Geometry check sheet. Reference: the model listing, model coordinates, mm. Face numbers are marked on the shaded views. A direction names the side the tool comes from. Give positions to 0.01 mm unless a question says otherwise; leave off trailing zeros. Write each loop counter-clockwise with the first axis right and the second up, starting at its lowest first coordinate (ties: lowest second). Pieces come first, ordered by that corner, then holes.
(1) Tool access check on the marked faces 1, 2, 3 and 4. Record the directions out of +Z, -Z, +X, -X, +Y, -Y that give a thin tool (end or side, any length) a straight path to the whole face; none if there is none.
(2) Cross-section at D-D (z = -2.5). Record the boundary of the cut face in (x, y) (3 decimals), and give its area (3 significant figures).
(3) Cross-section at C-C (y = -7.75). Record the boundary of the cut face in (x, z) (3 decimals).
(4) Cross-section at B-B (x = -2.4). Record the boundary of the cut face in (y, z) (3 decimals).
(5) Mould release check, pull along Z, two halves, no side actions. Record for the marked faces 5, 6 and 7: +Z half, -Z half, draft (parallel to the pull), parting line (faces both ways), or undercut.
(6) Thickness scan on line 1 along Z through (x, y) = (-2.5, -11) (3 decimals); line 2 along Z through (x, y) = (-13.6, -10.35) (3 decimals); line 3 along Z through (x, y) = (-5, -10.25) (3 decimals). Record the ranges inside material, lowest first.
(7) Depth check by flat-ended pin: P1, Ø1.3, axis at x = -8.5, y = 3.5, coming from the -Z side (3 decimals); P2, Ø5.5, axis at x = -13.6, z = 16.675, coming from the -Y side; P3, Ø2, axis at y = -1, z = -0.5, coming from the +X side; P4, Ø1, axis at x = -14.5, y = 2, coming from the +Z side (3 decimals). Enter the tip coordinate at first touch or a pass-through.
(8) Cross-section at A-A (y = -10.25). Record the boundary of the cut face in (x, z) (3 decimals).
Autodesk Inventor part; units mm, degrees
ref_plane "YZ Plane" through (0, 0, 0) normal (1, 0, 0) x (0, 1, 0)
ref_plane "XZ Plane" through (0, 0, 0) normal (0, 1, 0) x (-1, 0, 0)
ref_plane "XY Plane" through (0, 0, 0) normal (0, 0, 1) x (1, 0, 0)
sketch "Sketch1" plane through (0, 0, 0) normal (1, 0, 0) x (0, 1, 0)
  line L0 (2.5, 8) -> (-2.5, -8) construction
  line L1 (-2.5, 8) -> (2.5, -8) construction
  line L2 (2.5, 8) -> (2.5, 3.55)
  line L3 (2.5, -8) -> (2.5, -3.55)
  line L4 (-2.5, 0) -> (0.675, 0)
  line L5 (2.5, 8) -> (8.85, 8)
  line L6 (8.85, 8) -> (8.85, -8)
  line L7 (8.85, -8) -> (2.5, -8)
  arc A0 (2.5, -3.55) -> (2.5, 3.55) centre (0.675, 0) ccw
  line L8 (2.5, -8) -> (2.5, -3.55)
  line L9 (2.5, 3.55) -> (2.5, 8)
  point P0 (0, 0)
  dimension "d0" = 5
  dimension "d1" = 16
  dimension "d2" = 4.45
  dimension "d4" = 3.175
  dimension "d7" = 6.35
extrude "Extrusion1" add sketch "Sketch1" along normal blind 3.175
sketch "Sketch2" plane through (0, 0, 0) normal (-1, 0, 0) x (0, 0, 1)
  line L0 (-8, 8.85) -> (8, 8.85)
  line L1 (8, 2.5) -> (3.55, 2.5)
  line L2 (-8, 8.85) -> (8, 8.85)
  line L3 (8, 8.85) -> (8, 2.5)
  line L4 (8, 2.5) -> (-8, 2.5)
  line L5 (-8, 2.5) -> (-8, 8.85)
  point P0 (0, 0)
extrude "Extrusion2" add sketch "Sketch2" along normal blind 16
sketch "Sketch3" plane through (-16, 0, 0) normal (-1, 0, 0) x (0, 0, 1)
  line L0 (-8, 2.5) -> (-8, 8.85)
  line L1 (8, 2.5) -> (3.55, 2.5)
  line L2 (-8, 8.85) -> (8, 8.85)
  line L3 (8, 8.85) -> (8, 2.5)
  line L4 (8, 2.5) -> (-8, 2.5)
  line L5 (-8, 2.5) -> (-8, 8.85)
  point P0 (0, 0)
extrude "Extrusion3" add sketch "Sketch3" along normal blind 3.175
sketch "Sketch4" plane through (3.175, 2.5, 3.55) normal (0, -1, 0) x (1, 0, 0)
  line L0 (-22.35, -11.55) -> (-22.35, 4.45)
  line L1 (-3.175, -7.1) -> (0, -7.1)
  line L2 (-19.175, 0) -> (-3.175, 0)
  line L3 (-3.175, 0) -> (-3.175, -7.1)
  line L4 (-3.175, -7.1) -> (-19.175, -7.1)
  line L5 (-19.175, -7.1) -> (-19.175, 0)
  line L6 (-19.175, 0) -> (-3.175, -7.1) construction
  line L7 (-3.175, 0) -> (-19.175, -7.1) construction
  point P0 (-3.175, -3.55)
extrude "Extrusion4" cut sketch "Sketch4" against normal through all
sketch "Sketch5" plane through (-16, 2.5, 3.55) normal (1, 0, 0) x (0, 0, -1)
  line L0 (0, 6.35) -> (7.1, 6.35)
  line L1 (0, 0) -> (7.1, 0)
  line L2 (7.1, 0) -> (7.1, 6.35)
  line L3 (7.1, 6.35) -> (0, 6.35)
  line L4 (0, 6.35) -> (0, 0)
  point P0 (3.55, -2.5)
extrude "Extrusion5" cut sketch "Sketch5" against normal blind 0.25
sketch "Sketch6" plane through (0, 0.675, 0) normal (-1, 0, 0) x (0, 0, 1)
  line L0 (-3.55, 1.825) -> (-3.55, 8.175)
  line L1 (3.55, 1.825) -> (3.55, 8.175)
  line L2 (-3.55, 1.825) -> (3.55, 1.825)
  line L3 (3.55, 1.825) -> (3.55, 8.175)
  line L4 (3.55, 8.175) -> (-3.55, 8.175)
  line L5 (-3.55, 8.175) -> (-3.55, 1.825)
  point P0 (0, -0.675)
extrude "Extrusion6" cut sketch "Sketch6" against normal blind 0.25
sketch "Sketch7" plane through (3.175, 2.5, 8) normal (0, 0, 1) x (1, 0, 0)
  line L0 (-22.35, 6.35) -> (0, 6.35)
  line L1 (0, 6.35) -> (0, 0)
  line L2 (0, 0) -> (-22.35, 0)
  line L3 (-22.35, 0) -> (-22.35, 6.35)
  point P0 (-3.175, -2.5)
extrude "Extrusion7" add sketch "Sketch7" along normal blind 3.175
sketch "Sketch8" plane through (3.175, 2.5, -8) normal (0, 0, -1) x (-1, 0, 0)
  line L0 (0, 6.35) -> (22.35, 6.35)
  line L1 (22.35, 6.35) -> (22.35, 0)
  line L2 (0, 6.35) -> (22.35, 6.35)
  line L3 (22.35, 6.35) -> (22.35, 0)
  line L4 (22.35, 0) -> (0, 0)
  line L5 (0, 0) -> (0, 6.35)
  point P0 (3.175, -2.5)
extrude "Extrusion8" add sketch "Sketch8" along normal blind 3.175
sketch "Sketch9" plane through (-16.25, 2.5, -3.55) normal (0, -1, 0) x (1, 0, 0)
  line L0 (19.425, -7.625) -> (-2.925, -7.625)
  line L1 (-2.925, 14.725) -> (-2.925, -7.625)
  line L2 (19.425, -7.625) -> (-2.925, -7.625)
  line L3 (-2.925, -7.625) -> (-2.925, -4.45)
  line L4 (-2.925, -4.45) -> (19.425, -4.45)
  line L5 (19.425, -4.45) -> (19.425, -7.625)
  line L6 (19.425, 7.1) -> (19.425, 14.725)
  line L7 (-2.925, 14.725) -> (19.425, 14.725)
  line L8 (19.425, 14.725) -> (19.425, 11.55)
  line L9 (19.425, 11.55) -> (-2.925, 11.55)
  line L10 (-2.925, 11.55) -> (-2.925, 14.725)
  point P0 (16.25, 3.55)
  dimension "d26" = 3.175
  dimension "d27" = 3.175
extrude "Extrusion9" add sketch "Sketch9" along normal blind 15.142
sketch "Sketch10" plane through (3.175, 2.5, 11.175) normal (0, 0, 1) x (1, 0, 0)
  line L0 (0, -15.142) -> (-22.35, -15.142)
  line L1 (0, 0) -> (0, -15.142)
  line L2 (-22.35, -15.142) -> (0, -15.142)
  line L3 (0, -15.142) -> (0, -11.967)
  line L4 (0, -11.967) -> (-22.35, -11.967)
  line L5 (-22.35, -11.967) -> (-22.35, -15.142)
  point P0 (-3.175, -2.5)
  dimension "d30" = 3.175
extrude "Extrusion10" add sketch "Sketch10" along normal blind 5.715
sketch "Sketch11" plane through (3.175, 2.5, -11.175) normal (0, 0, -1) x (-1, 0, 0)
  line L0 (22.35, -15.142) -> (0, -15.142)
  line L1 (22.35, 0) -> (22.35, -15.142)
  line L2 (0, -15.142) -> (22.35, -15.142)
  line L3 (22.35, -15.142) -> (22.35, -11.967)
  line L4 (22.35, -11.967) -> (0, -11.967)
  line L5 (0, -11.967) -> (0, -15.142)
  point P0 (3.175, -2.5)
  dimension "d33" = 3.175
extrude "Extrusion11" add sketch "Sketch11" along normal blind 5.715
chamfer "Chamfer1" [suppressed]
sketch "Sketch14" plane through (3.175, 2.5, 16.89) normal (0, 0, 1) x (1, 0, 0)
  line L0 (0, -11.967) -> (-22.35, -11.967)
  line L1 (0, 0) -> (0, -15.142)
  line L2 (-22.35, -11.967) -> (0, -11.967)
  line L3 (0, -11.967) -> (0, -15.142)
  line L4 (0, -15.142) -> (-22.35, -15.142)
  line L5 (-22.35, -15.142) -> (-22.35, -11.967)
  point P0 (-3.175, -2.5)
extrude "Extrusion12" add sketch "Sketch14" along normal blind 5.285
sketch "Sketch15" plane through (3.175, 2.5, -16.89) normal (0, 0, -1) x (-1, 0, 0)
  line L0 (0, -11.967) -> (0, -15.142)
  line L1 (0, -15.142) -> (22.35, -15.142)
  line L2 (0, -11.967) -> (22.35, -11.967)
  line L3 (22.35, -11.967) -> (22.35, -15.142)
  line L4 (22.35, -15.142) -> (0, -15.142)
  line L5 (0, -15.142) -> (0, -11.967)
  point P0 (3.175, -2.5)
extrude "Extrusion13" add sketch "Sketch15" along normal blind 5.285
sketch "Sketch16" plane through (-19.175, -9.467, -11.175) normal (0, 1, 0) x (1, 0, 0)
  point P0 (19.175, -11.175)
chamfer "Chamfer2" distance 3 angle 45 2 edges at (-8, 8.85, 11.175) (-8, 8.85, -11.175)
sketch "Sketch20" plane through (-19.175, 2.5, -8) normal (0, 0, 1) x (1, 0, 0)
  line L0 (0, -15.142) -> (22.35, -15.142)
  line L1 (22.35, -15.142) -> (22.35, 0)
  line L2 (22.35, 0) -> (0, 0)
  line L3 (0, 0) -> (0, -15.142)
  point P0 (19.175, -2.5)
extrude "Extrusion17" cut sketch "Sketch20" against normal blind 0.125
sketch "Sketch21" plane through (3.175, 2.5, 8) normal (0, 0, -1) x (-1, 0, 0)
  line L0 (22.35, 0) -> (22.35, -15.142)
  line L1 (0, 0) -> (0, -15.142)
  line L2 (22.35, -15.142) -> (0, -15.142)
  line L3 (0, -15.142) -> (0, 0)
  line L4 (0, 0) -> (22.35, 0)
  line L5 (22.35, 0) -> (22.35, -15.142)
  point P0 (3.175, -2.5)
  point P1 (0, -15.142)
extrude "Extrusion18" cut sketch "Sketch21" against normal blind 0.125
sketch "Sketch22" plane through (-19.175, 8.85, -8.175) normal (0, 1, 0) x (1, 0, 0)
  line L0 (19.425, -11.725) -> (22.35, -11.725)
  line L1 (19.425, -4.625) -> (22.35, -4.625)
  line L2 (19.425, -11.725) -> (22.35, -11.725)
  line L3 (22.35, -11.725) -> (22.35, -4.625)
  line L4 (22.35, -4.625) -> (19.425, -4.625)
  line L5 (19.425, -4.625) -> (19.425, -11.725)
  point P0 (19.175, -8.175)
extrude "Extrusion19" cut sketch "Sketch22" against normal through all
sketch "Sketch23" plane through (-19.175, -9.467, 11.175) normal (0, 1, 0) x (1, 0, 0)
  line L0 (0, 0) -> (0, -11)
  line L1 (22.35, 0) -> (22.35, -11)
  point P0 (19.175, 11.175)
  point P1 (5.575, -5.5)
  point P2 (16.775, -5.5)
sketch "Sketch24" plane through (-19.175, -9.467, -11.175) normal (0, 1, 0) x (1, 0, 0)
  line L0 (22.35, 0) -> (22.35, 11)
  line L1 (0, 0) -> (0, 11)
  point P0 (19.175, -11.175)
  point P1 (16.775, 5.5)
  point P2 (5.575, 5.5)
hole "Hole1" at (-13.6, -9.467, -16.675) direction (0, -1, 0) diameter 3.454 end through all
hole "Hole2" at (-2.4, -9.467, -16.675) direction (0, -1, 0) diameter 3.454 end through all
hole "Hole3" at (-2.4, -9.467, 16.675) direction (0, -1, 0) diameter 3.454 end through all
hole "Hole4" at (-13.6, -9.467, 16.675) direction (0, -1, 0) diameter 3.454 end through all
sketch "Sketch25" plane through (3.175, 0, 0) normal (1, 0, 0) x (0, 0, -1)
  line L0 (3.55, 5.0908) -> (8.175, 5.0908)
  line L1 (8.175, 8.85) -> (-8.175, 8.85)
  line L2 (8.175, 5.0908) -> (8.175, 8.85)
  line L3 (8.175, 8.85) -> (3.55, 8.85)
  line L4 (3.55, 8.85) -> (8.175, 8.85)
  line L5 (8.175, 8.85) -> (8.175, 5.0908)
  line L6 (8.175, 5.0908) -> (3.55, 5.0908)
  line L7 (3.55, 5.0908) -> (3.55, 8.85)
  point P0 (0, 0)
  point P1 (3.55, 2.5)
  dimension "d102" = 2.5908
extrude "Extrusion20" [suppressed]
chamfer "Chamfer3" [suppressed]
sketch "Sketch26" plane through (3.175, 0, 0) normal (1, 0, 0) x (0, 0, -1)
  line L0 (3.55, 2.5) -> (-3.55, 2.5)
  line L1 (-3.55, 2.5) -> (-3.55, 5.675)
  line L2 (-3.55, 2.5) -> (-3.55, 8.85)
  line L3 (-3.55, 5.675) -> (-11.175, 5.675)
  line L4 (-11.175, 5.85) -> (-11.175, -9.467)
  line L5 (-11.175, 5.85) -> (-8.175, 8.85)
  line L6 (-8.175, 8.85) -> (-3.55, 8.85)
  line L7 (3.55, 8.85) -> (3.55, 2.5)
  line L8 (3.55, 2.5) -> (3.55, 5.675)
  line L9 (3.55, 5.675) -> (11.175, 5.675)
  line L10 (11.175, 5.85) -> (11.175, -9.467)
  line L11 (11.175, 5.85) -> (8.175, 8.85)
  line L12 (11.175, 5.85) -> (8.175, 8.85)
  line L13 (8.175, 8.85) -> (3.55, 8.85)
  line L14 (3.55, 8.85) -> (3.55, 5.675)
  point P0 (0, 0)
  dimension "d109" = 3.175
  dimension "d110" = 3.175
extrude "Extrusion21" cut sketch "Sketch26" against normal through all
sketch "Sketch27" plane through (-19.175, 8.85, -3.55) normal (0, 1, 0) x (1, 0, 0)
  line L0 (2.925, 0) -> (2.925, -7.1)
  line L1 (0, 0) -> (2.925, 0)
  line L2 (2.925, 0) -> (2.925, -7.1)
  line L3 (2.925, -7.1) -> (0, -7.1)
  line L4 (0, -7.1) -> (0, 0)
  point P0 (19.175, -3.55)
extrude "Extrusion22" cut sketch "Sketch27" against normal blind 3.175
sketch "Sketch28" plane through (-16.25, 2.5, -3.55) normal (0, -1, 0) x (1, 0, 0)
  line L0 (-2.925, 11.675) -> (-2.925, -4.575)
  line L1 (-2.925, -4.575) -> (19.425, -4.575)
  line L2 (-2.925, 11.675) -> (0, 11.675)
  line L3 (0, 11.675) -> (0, -4.575)
  line L4 (0, -4.575) -> (-2.925, -4.575)
  line L5 (-2.925, -4.575) -> (-2.925, 11.675)
  point P0 (16.25, 3.55)
  dimension "d115" = 2.925
extrude "Extrusion23" add sketch "Sketch28" along normal blind 3.175
chamfer "Chamfer4" [suppressed]
sketch "Sketch29" plane through (-16.25, -12.642, -3.55) normal (0, -1, 0) x (1, 0, 0)
  line L0 (-2.925, 11.675) -> (19.425, 11.675)
  line L1 (19.425, -4.575) -> (-2.925, -4.575)
  line L2 (19.425, 11.675) -> (-2.925, 11.675)
  line L3 (-2.925, 11.675) -> (-2.925, -4.575)
  line L4 (-2.925, -4.575) -> (19.425, -4.575)
  line L5 (19.425, -4.575) -> (19.425, 11.675)
  point P0 (16.25, 3.55)
extrude "Extrusion24" [suppressed]
sketch "Sketch30" plane through (-16.25, -12.642, -3.55) normal (0, -1, 0) x (1, 0, 0)
  line L0 (-2.925, 11.675) -> (19.425, 11.675)
  line L1 (-2.925, -4.575) -> (-2.925, -18.625)
  line L2 (19.425, 11.675) -> (-2.925, 11.675)
  line L3 (-2.925, 11.675) -> (-2.925, -4.575)
  line L4 (-2.925, -4.575) -> (19.425, -4.575)
  line L5 (19.425, -4.575) -> (19.425, 11.675)
  point P0 (16.25, 3.55)
extrude "Extrusion25" [suppressed]
sketch "Sketch31" plane through (3.175, 5.675, 11.175) normal (0, 1, 0) x (1, 0, 0)
  line L0 (-19.425, 14.725) -> (-19.425, 7.625)
  line L1 (0, 14.725) -> (-19.425, 14.725)
  line L2 (-19.425, 14.725) -> (-19.425, 7.625)
  line L3 (-19.425, 7.625) -> (0, 7.625)
  line L4 (-19.425, 7.625) -> (0, 7.625)
  line L5 (0, 7.625) -> (0, 0)
  line L6 (0, 0) -> (-22.35, 0)
  line L7 (0, 0) -> (-22.35, 0)
  line L8 (-22.35, 0) -> (-22.35, 22.35)
  line L9 (-22.35, 0) -> (-22.35, 22.35)
  line L10 (-22.35, 22.35) -> (0, 22.35)
  line L11 (0, 22.35) -> (0, 14.725)
  point P0 (-3.175, 11.175)
extrude "Extrusion26" cut sketch "Sketch31" against normal blind 0.5
sketch "Sketch32" plane through (3.175, 5.175, 11.175) normal (0, 1, 0) x (1, 0, 0)
  line L0 (0, 22.35) -> (-22.35, 22.35)
  line L1 (-22.35, 0) -> (0, 0)
  line L2 (-22.35, 22.35) -> (0, 22.35)
  line L3 (0, 22.35) -> (0, 0)
  line L4 (0, 0) -> (-22.35, 0)
  line L5 (-22.35, 0) -> (-22.35, 22.35)
  point P0 (-3.175, 11.175)
extrude "Extrusion27" cut sketch "Sketch32" against normal blind 1.075
sketch "Sketch33" plane through (3.175, 2.5, 11.175) normal (0, 0, 1) x (1, 0, 0)
  line L0 (-22.35, 1.6) -> (0, 1.6)
  line L1 (0, -11.967) -> (0, -15.142)
  line L2 (-22.35, 1.6) -> (0, 1.6)
  line L3 (0, 1.6) -> (0, -11.967)
  line L4 (0, -11.967) -> (-22.35, -11.967)
  line L5 (-22.35, -11.967) -> (-22.35, 1.6)
  point P0 (-3.175, -2.5)
extrude "Extrusion28" cut sketch "Sketch33" against normal blind 1.45
sketch "Sketch34" plane through (3.175, 2.5, -11.175) normal (0, 0, -1) x (-1, 0, 0)
  line L0 (0, -11.967) -> (22.35, -11.967)
  line L1 (22.35, 1.6) -> (0, 1.6)
  line L2 (22.35, -11.967) -> (0, -11.967)
  line L3 (0, -11.967) -> (0, 1.6)
  line L4 (0, 1.6) -> (22.35, 1.6)
  line L5 (22.35, 1.6) -> (22.35, -11.967)
  point P0 (3.175, -2.5)
extrude "Extrusion29" cut sketch "Sketch34" against normal blind 1.45
fillet "Fillet1" radius 3 2 edges at (-8, -9.467, 9.725) (-8, -9.467, -9.725)
fillet "Fillet2" radius 2 2 edges at (-17.7125, -0.675, -8.125) (-17.7125, -0.675, 8.125)
properties part number "peltierclip_ledgereod2"
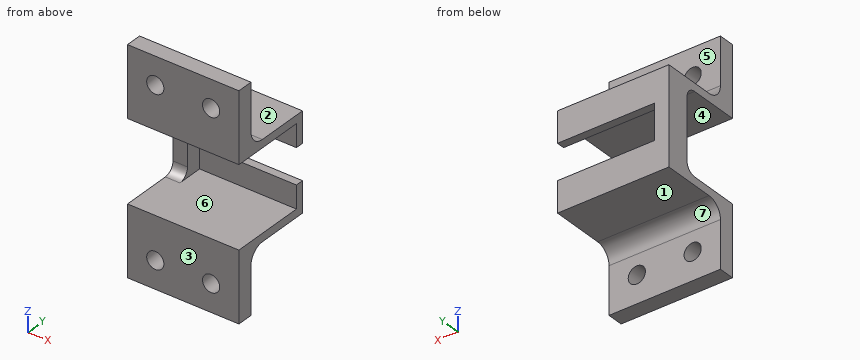
Reply:
1. face 1: -Z, +X, -X, +Y
1. face 2: +Z, +X, -X, +Y
1. face 3: +Z, -Z, +X, -X, -Y
1. face 4: +X, -Y
2. outline: (-19.175, -0.675) - (-16.25, -0.675) - (-16.25, 4.1) - (-19.175, 4.1) - close
2. area: 14.0 mm2
3. outline: (-19.175, -10.013) - (3.175, -10.013) - (3.175, -8.125) - (-19.175, -8.125) - close; (-19.175, 8.125) - (3.175, 8.125) - (3.175, 10.013) - (-19.175, 10.013) - close
4. outline: (-12.642, -22.175) - (-9.467, -22.175) - (-9.467, -18.402) - (-12.642, -18.402) - close; (-12.642, -14.948) - (-9.467, -14.948) - (-9.467, -12.725) arc R3 cw to (-6.467, -9.725) - (4.1, -9.725) - (4.1, -3.55) - (2.5, -3.55) - (2.5, -8.125) - (-12.642, -8.125) - close; (-12.642, 8.125) - (2.5, 8.125) - (2.5, 3.55) - (4.1, 3.55) - (4.1, 9.725) - (-6.467, 9.725) arc R3 cw to (-9.467, 12.725) - (-9.467, 14.948) - (-12.642, 14.948) - close; (-12.642, 18.402) - (-9.467, 18.402) - (-9.467, 22.175) - (-12.642, 22.175) - close
5. face 5: draft
5. face 6: undercut
5. face 7: -Z half
6. line 1: z = -22.175 to -18.399, -14.951 to -8.125, 8.125 to 14.951, 18.399 to 22.175
6. line 2: z = -22.175 to -18.402, -14.948 to -8.125, 8.125 to 14.948, 18.402 to 22.175
6. line 3: z = -22.175 to -8.125, 8.125 to 22.175
7. P1: stops at z = -9.725
7. P2: stops at y = -12.64
7. P3: stops at x = -16.25
7. P4: stops at z = 9.725
8. outline: (-19.175, -22.175) - (3.175, -22.175) - (3.175, -8.125) - (-19.175, -8.125) - close; (-19.175, 8.125) - (3.175, 8.125) - (3.175, 22.175) - (-19.175, 22.175) - close; hole circle Ø3.454 at (-13.6, -16.675); hole circle Ø3.454 at (-13.6, 16.675); hole circle Ø3.454 at (-2.4, -16.675); hole circle Ø3.454 at (-2.4, 16.675)
